```python
from build123d import *

# Parameters (mm, degrees)
F1_W     = 40
F1_H     = 33
F3_DEPTH = 1240
F2_W     = 80
F2_H     = 100
F4_DEPTH = 25
F5_W     = 2480
F5_H     = 50
F6_DEPTH = 2512


# Not quite as in the source:
# - an extrude ends at something that could not be found from the text; its depth is read off the source's solid


with BuildPart() as f3:
    # F1 (on Right) → F3 (new body, symmetric)
    with BuildSketch(Plane.YZ):
        Polygon((20, 33), (20, 63), (17, 66), (12, 66), (12, 80), (4, 80), (4, 66), (-4, 66), (-4, 80), (-12, 80), (-12, 66), (-17, 66), (-20, 63), (-20, 33), align=None)
        with Locations((0, 16.5)):
            Rectangle(F1_W, F1_H)
        with Locations((0, -16.5)):
            Rectangle(F1_W, F1_H)
    extrude(amount=F3_DEPTH, both=True)

    # F2 (on Front) → F4 (cut, symmetric)
    with BuildSketch(Plane.XZ):
        with Locations((-1240, 83)):
            Rectangle(F2_W, F2_H)
        with Locations((-1240, -83)):
            Rectangle(F2_W, F2_H)
    extrude(amount=F4_DEPTH, both=True, mode=Mode.SUBTRACT)

    # F5 (on face) → F6 (cut, through all)
    with BuildSketch(Plane.XZ.offset(20)):
        with Locations((0, -58)):
            Rectangle(F5_W, F5_H)
    extrude(amount=-F6_DEPTH, mode=Mode.SUBTRACT)


solid = f3.part
```
Part model, mm, in its own coordinate system. A direction names the side the tool comes from. Round coordinates to 2 decimals unless told otherwise and drop trailing zeros. Write each loop counter-clockwise with the first axis right and the second up, starting at its lowest first coordinate (ties: lowest second). Pieces come first, ordered by that corner, then holes. Notation, with made-up numbers: (18, 42.5) -> (33, 42.5) arc R31 cw to (33, 78.5) -> close; hole circle Ø5 at (82.25, 86). An arc over 180 degrees is marked (long way). Return JSON: item names as keys, results as strings. Group by question number.
Q1. Which spindle directions (+Z, -Z, +X, -X, +Y, -Y) get a long thin tool onto all of the face, cutting with end or side? Do faces 1 (the flat face through (-1220, 0, 33)), 2 (the flat face through (-1240, 0, 0)). Say none if no direction does.
Q2. Pin check, flat tips, straight feed: pin 1 (15.5 mm diameter, centred on x = 622.5, z = 75.5, fed in from -Y); pin 2 (4 mm diameter, centred on x = -90, z = 74.5, fed in from +Y); pin 3 (4 mm diameter, centred on x = -276, y = -1.5, fed in from +Z). Stop position of each tip, or through.
Q3. Saw through at A-A on x = -772.5. Write the cut outline in (y, z).
Q4. Probe L1, parallel to Z at x = -478.5, y = 3.5; L2, parallel to Y at x = 1115, z = 72.5; L3, parallel to X at y = 5, z = 51.5. List the from-to ranges inside material, lowest first. Write a range as [from, to].
Answer:
{
 "1": {"face 1": "+Z, -X, +Y, -Y", "face 2": "+Z, -Z, -X, +Y, -Y"},
 "2": {"pin 1": "y = -12", "pin 2": "y = 12", "pin 3": "z = 66"},
 "3": {"outline": "(-20, -33) -> (20, -33) -> (20, 63) -> (17, 66) -> (12, 66) -> (12, 80) -> (4, 80) -> (4, 66) -> (-4, 66) -> (-4, 80) -> (-12, 80) -> (-12, 66) -> (-17, 66) -> (-20, 63) -> close"},
 "4": {"L1": "[-33, 66]", "L2": "[-12, -4], [4, 12]", "L3": "[-1200, 1240]"}
}
